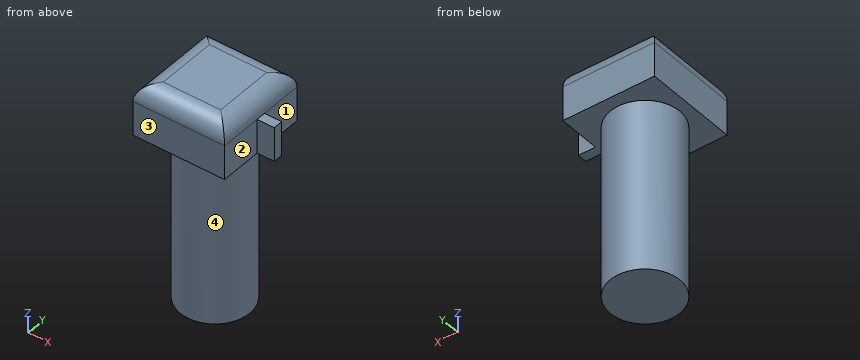
```python
from build123d import *

# Parameters (mm, degrees)
F0_R     = 51.425526
F1_DEPTH = 254
F2_W     = 135.8829
F2_H     = 139.160782
F3_DEPTH = 76.2
F4_R     = 25.4
F5_W     = 14.30345
F5_H     = 50.8
F6_DEPTH = 25.4


with BuildPart() as f1:
    # F0 (on Top) → F1 (new body)
    with BuildSketch(Plane.XY):
        Circle(F0_R)
    extrude(amount=F1_DEPTH)

    # F2 (on face) → F3 (join)
    with BuildSketch(Plane.XY.offset(254)):
        Rectangle(F2_W, F2_H)
    extrude(amount=F3_DEPTH)

    # F4
    f4_edges = [f1.edges().sort_by_distance(p)[0] for p in [
        (67.94145, 0, 330.2),
        (0, 69.580391, 330.2),
        (-67.94145, 0, 330.2),
        (0, -69.580391, 330.2),
    ]]
    fillet(f4_edges, radius=F4_R)

    # F5 (on face) → F6 (join)
    with BuildSketch(Plane.YZ.offset(67.94145)):
        with Locations((0, 279.4)):
            Rectangle(F5_W, F5_H)
    extrude(amount=F6_DEPTH)


solid = f1.part
```
Verification items for the finished model (mm, model axes). Face numbers are marked on the shaded views. A direction names the side the tool comes from. Round coordinates to 2 decimals unless told otherwise and drop trailing zeros. Order: outer loops, then holes, each group sorted by start corner. A loop starts at its lowest first (then second) coordinate and runs counter-clockwise, first axis right, second up. Notation, with made-up numbers: (16, 20.5) -> (69, 20.5) arc R20 cw to (69, 39.5) -> close; hole circle Ø7 at (49.25, 5). An arc over 180 degrees is marked (long way). Put each result on its own line as item: value. Start each with the question number.
(1) Depth check by flat-ended pin: pin 1 Ø3 at (x, z) = (-31.5, 195.5) entering from +Y; pin 2 Ø12.5 at (x, z) = (76, 291.5) entering from -Y; pin 3 Ø3 at (y, z) = (43.5, 205.5) entering from +X. Enter the tip coordinate at first touch or a pass-through.
(2) Material ranges on line 1 along Z through (x, y) = (-43, -18.5); line 2 along X through (y, z) = (-31, 273); line 3 along Z through (x, y) = (-14.5, 59), recorded low to high.
(3) Tool access check on the marked faces 1, 2, 3 and 4. Record the directions out of +Z, -Z, +X, -X, +Y, -Y that give a thin tool (end or side, any length) a straight path to the whole face; none if there is none.
(4) Section check A-A (z = 277). Enter the section's corners in (x, y).
(5) Section check B-B (y = 0). Enter the section's corners in (x, z).
(6) Section check D-D (y = 26). Enter the section's corners in (x, z), then the cut area to 3 significant figures.
(7) Section check C-C (x = 0). Enter the section's corners in (y, z).
Completed:
1. pin 1: stops at y = 41.77
1. pin 2: stops at y = -7.15
1. pin 3: stops at x = 29.67
2. line 1: z = 0 to 330.2
2. line 2: x = -67.94 to 67.94
2. line 3: z = 254 to 325.43
3. face 1: +Z, -Z, +X, +Y
3. face 2: +Z, -Z, +X, -Y
3. face 3: +Z, -Z, +X, -X, -Y
3. face 4: -Z
4. outline: (-67.94, -69.58) -> (67.94, -69.58) -> (67.94, -7.15) -> (93.34, -7.15) -> (93.34, 7.15) -> (67.94, 7.15) -> (67.94, 69.58) -> (-67.94, 69.58) -> close
5. outline: (-67.94, 254) -> (-51.43, 254) -> (-51.43, 0) -> (51.43, 0) -> (51.43, 254) -> (93.34, 254) -> (93.34, 304.8) -> (67.94, 304.8) arc R25.4 ccw to (42.54, 330.2) -> (-42.54, 330.2) arc R25.4 ccw to (-67.94, 304.8) -> close
6. outline: (-67.94, 254) -> (-44.37, 254) -> (-44.37, 0) -> (44.37, 0) -> (44.37, 254) -> (67.94, 254) -> (67.94, 304.8) arc R25.4 ccw to (42.54, 330.2) -> (-42.54, 330.2) arc R25.4 ccw to (-67.94, 304.8) -> close
6. area: 32,600 mm2
7. outline: (-69.58, 254) -> (-51.43, 254) -> (-51.43, 0) -> (51.43, 0) -> (51.43, 254) -> (69.58, 254) -> (69.58, 304.8) arc R25.4 ccw to (44.18, 330.2) -> (-44.18, 330.2) arc R25.4 ccw to (-69.58, 304.8) -> close
